from build123d import *

# Parameters (mm, degrees)
SKETCH1_W   = 187.96
SKETCH1_H   = 23.368
BASE_DEPTH  = 5.334
SKETCH3_W   = 25.4
SKETCH3_H   = 5.334
SKETCH3_W_2 = 38.1
SKETCH3_W_3 = 107.95
TABS_DEPTH  = 190.482127337
SKETCH4_R   = 2.9718
AXLE_DEPTH  = 190.482127337


with BuildPart() as part:
    # Sketch1 → Base (new body)
    with BuildSketch(Plane(origin=(0, 0, 0), x_dir=(0, 0, -1), z_dir=(1, 0, 0))):
        with Locations((93.98, 11.684)):
            Rectangle(SKETCH1_W, SKETCH1_H)
    extrude(amount=BASE_DEPTH)

    # Sketch3 → Tabs (cut, through all)
    with BuildSketch(Plane(origin=(5.334, 0, 0), x_dir=(0, 0, -1), z_dir=(1, 0, 0))):
        with Locations((48.26, 20.701)):
            Rectangle(SKETCH3_W, SKETCH3_H)
        with Locations((111.76, 2.667)):
            Rectangle(SKETCH3_W_2, SKETCH3_H)
        with Locations((168.91, 2.667)):
            Rectangle(SKETCH3_W_2, SKETCH3_H)
        with Locations((133.985, 20.701)):
            Rectangle(SKETCH3_W_3, SKETCH3_H)
    extrude(amount=-TABS_DEPTH, mode=Mode.SUBTRACT)

    # Sketch4 → Axle (cut, through all)
    with BuildSketch(Plane(origin=(5.334, 0, 0), x_dir=(0, 0, -1), z_dir=(1, 0, 0))):
        with Locations((12.7, 11.684)):
            Circle(SKETCH4_R)
    extrude(amount=-AXLE_DEPTH, mode=Mode.SUBTRACT)


solid = part.part
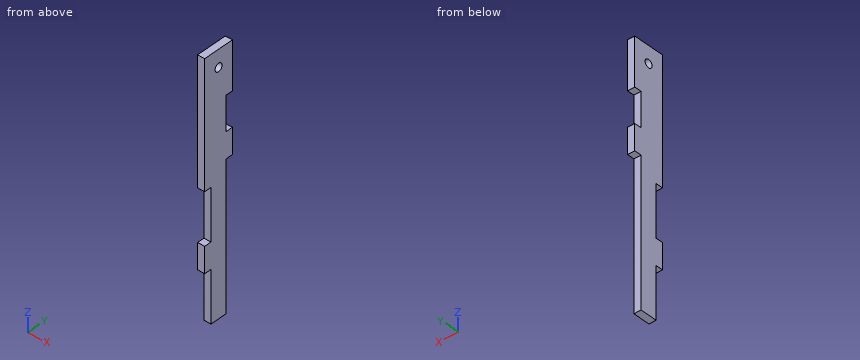
The model under review builds one solid part; all positions refer to its coordinate system, in mm. Round coordinates to 2 decimals unless told otherwise and drop trailing zeros. Loops run counter-clockwise (first coordinate to the right, second up) from the corner with the lowest first, then second, coordinate; pieces in that order, holes last. Notation, with made-up numbers: M -22.75,-1 L 21.25,-1 A23 cw 21.25,36 Z; hole C 36.25,-17 d2. An arc over 180 degrees is marked long. Answer as CSV lines item,"result".
1. To check wall thickness, follow L1, parallel to Y at x = 2.5, z = -12.7; L2, parallel to Z at x = 1.35, y = 4.75; L3, parallel to Z at x = 5, y = 19.25. State the ranges of each line that lie inside material, in increasing order. Write a range as [from, to].
Outcome:
L1,"y = [0, 8.71], [14.66, 23.37]"
L2,"z = [-149.86, -130.81], [-92.71, 0]"
L3,"z = [-80.01, -60.96], [-35.56, 0]"
2. We need section B-B (y = 2.25). Give the boundary of the cut face in (x, z), plus the area to 3 significant figures.
Outcome:
outline,"M 0,-149.86 L 5.33,-149.86 L 5.33,-130.81 L 0,-130.81 Z; M 0,-92.71 L 5.33,-92.71 L 5.33,0 L 0,0 Z"
area,"596 mm2"
3. We need section D-D (z = -101). Give the boundary of the cut face in (x, y).
Outcome:
outline,"M 0,5.33 L 5.33,5.33 L 5.33,18.03 L 0,18.03 Z"
4. Insertion check: pin 1 Ø1 at (x, y) = (1, 2.5) entering from -Z; pin 2 Ø2.5 at (x, z) = (2, -127.5) entering from +Y; pin 3 Ø1.6 at (x, z) = (3, -170) entering from -Y; pin 4 Ø5.5 at (y, z) = (11.684, -12.7) entering from +X. Each pin has a flat end and moves straight along its axis. Give the tip position at first contact, or say it passes through.
Outcome:
pin 1,"stops at z = -149.86"
pin 2,"stops at y = 18.03"
pin 3,"stops at y = 5.33"
pin 4,"passes through"
5. We need section C-C (x = 2.1). Give the boundary of the cut face in (y, z), plus the area to 3 significant figures.
Outcome:
outline,"M 0,-149.86 L 5.33,-149.86 L 5.33,-187.96 L 18.03,-187.96 L 18.03,-80.01 L 23.37,-80.01 L 23.37,-60.96 L 18.03,-60.96 L 18.03,-35.56 L 23.37,-35.56 L 23.37,0 L 0,0 L 0,-92.71 L 5.33,-92.71 L 5.33,-130.81 L 0,-130.81 Z; hole C 11.68,-12.7 d5.94"
area,"3,250 mm2"
6. We need section A-A (z = -12.7). Give the boundary of the cut face in (x, y), plus the area to 3 significant figures.
Outcome:
outline,"M 0,0 L 5.33,0 L 5.33,8.71 L 0,8.71 Z; M 0,14.66 L 5.33,14.66 L 5.33,23.37 L 0,23.37 Z"
area,"92.9 mm2"
